The figure shows three views and two pictorial views of one solid part (mm, origin at its lowest corner). Answer the questions. Coordinates: 2 decimals unless noted, no trailing zeros. Write each loop counter-clockwise with the first axis right and the second up, starting at its lowest first coordinate (ties: lowest second). Pieces come first, ordered by that corner, then holes.
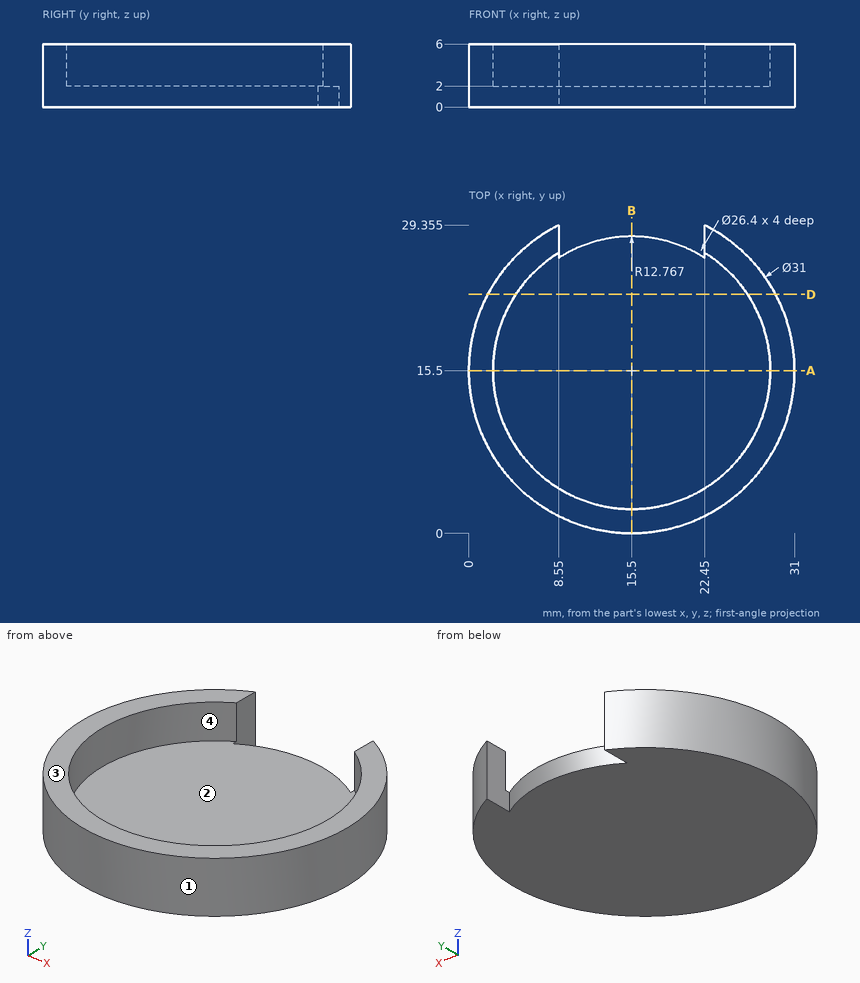
Q1. Determine the mould class of the marked faces 1, 2, 3 and 4 for opening direction X: released by +X, released by -X, zero draft, split by the parting line, or undercut.
Answers below:
face 1: split by the parting line
face 2: undercut
face 3: zero draft
face 4: undercut
Q2. The part is cut by section D-D, the plane y = 22.75. Write down the section's boundary in (x, z).
Answers below:
outline: (1.8, 0) - (29.2, 0) - (29.2, 6) - (26.53, 6) - (26.53, 2) - (4.47, 2) - (4.47, 6) - (1.8, 6) - close
Q3. Find the intervals of material crossed by probe 1 along X at (y, z) = (15.5, 2.9); probe 2 along Z at (x, y) = (8.5, 17.5); probe 3 along X at (y, z) = (18.5, 2.85) (1 decimal), in increasing order.
Answers below:
probe 1: x = 0 to 2.3, 28.7 to 31
probe 2: z = 0 to 2
probe 3: x = 0.3 to 2.6, 28.4 to 30.7
Q4. The part is cut by section A-A, the plane y = 15.5. Write down the section's boundary in (x, z).
Answers below:
outline: (0, 0) - (31, 0) - (31, 6) - (28.7, 6) - (28.7, 2) - (2.3, 2) - (2.3, 6) - (0, 6) - close
Q5. Given pin 1 (0.9 mm diameter, centred on y = 28, z = 2, fed in from -X); pin 2 (3.5 mm diameter, centred on y = 27.5, z = 3.5, fed in from +X); pin 3 (3 mm diameter, centred on x = 17, z = 2.5, fed in from +Y), each flat-ended and moving along its own axis, determine where each tip first touches the part or whether it passes through.
Answers below:
pin 1: stops at x = 5.75
pin 2: stops at x = 27.13
pin 3: stops at y = 28.27
Q6. The part is cut by section B-B, the plane x = 15.5. Write down the section's boundary in (y, z).
Answers below:
outline: (0, 0) - (28.27, 0) - (28.27, 2) - (2.3, 2) - (2.3, 6) - (0, 6) - close
